Geometry check sheet. Reference: the model listing, model coordinates, mm. A direction names the side the tool comes from. Coordinates: 2 decimals unless noted, no trailing zeros.
from build123d import *

# Parameters (mm, degrees)
ESQUISSE1_W                  = 20
ESQUISSE1_H                  = 18
BOSS_EXTRU_1_DEPTH           = 20
ENL_V_MAT_EXTRU_1_DEPTH      = 34.526109228
ENL_V_MAT_EXTRU_1_DEPTH_BACK = 34.526109228
ESQUISSE4_W                  = 23.372047651
ESQUISSE4_H                  = 17.8
ENL_V_MAT_EXTRU_3_DEPTH      = 1
CONG_2_R                     = 40
ESQUISSE5_R                  = 2.15
ENL_V_MAT_EXTRU_4_DEPTH      = 31.724582991
CONG_3_R                     = 9
CHANFREIN1_SIZE              = 20.578216064
CHANFREIN1_SIZE_2            = 4
CONG_4_R                     = 4
ESQUISSE6_R                  = 1.1
ENL_V_MAT_EXTRU_5_DEPTH      = 253.375332695
ESQUISSE10_R                 = 1.9
ENL_V_MAT_EXTRU_6_DEPTH      = 7.5


# Some blends are built 0.0001 mm under size
with BuildPart() as part:
    # Esquisse1 → Boss.-Extru.1 (new body)
    with BuildSketch(Plane.XY):
        with Locations((10, 3)):
            Rectangle(ESQUISSE1_W, ESQUISSE1_H)
    extrude(amount=BOSS_EXTRU_1_DEPTH)

    # Esquisse2 → Enlèv. mat.-Extru.1 (cut, two sides: drawn at the far end of the back side and taken through both)
    with BuildSketch(Plane(origin=(0, 12, 0), x_dir=(1, 0, 0), z_dir=(0, 1, 0)).offset(-ENL_V_MAT_EXTRU_1_DEPTH_BACK)):
        Polygon((85.451214086, 12.384445057), (20.045630921, -0.0408989), (0, -3.849042594), (0, 0), (0, 66.575366927), (71.310016401, 179.020907021), (156.761230487, 124.829985151), align=None)
    extrude(amount=ENL_V_MAT_EXTRU_1_DEPTH + ENL_V_MAT_EXTRU_1_DEPTH_BACK, mode=Mode.SUBTRACT)

    # Esquisse4 → Enlèv. mat.-Extru.3 (cut)
    with BuildSketch(Plane(origin=(0.705746644, 0, 3.714969257), x_dir=(-0.9824291803850712, 0, 0.1866357562952965), z_dir=(-0.1866357562952965, 0, -0.9824291803850712))):
        with Locations((-7.953308699, 3)):
            Rectangle(ESQUISSE4_W, ESQUISSE4_H)
    extrude(amount=-ENL_V_MAT_EXTRU_3_DEPTH, mode=Mode.SUBTRACT)

    # Congé2
    # the kernel refuses this fillet: 40 mm, written as the material it adds along each edge
    with BuildSketch(Plane(origin=(41.830053891, 11.9, -3.079684565), x_dir=(0, -1, 0), z_dir=(-0.9824291803850712, 0, 0.1866357562952965))) as cong_2_piece_1_section:
        with BuildLine():
            CenterArc((8.888194417, -40), CONG_2_R, 90, 12.838568141)
            Line((0, -1), (0, 0))
            Line((0, 0), (8.888194417, 0))
        make_face()
    cong_2_piece_1 = extrude(amount=64.798673587, mode=Mode.PRIVATE)
    cong_2_piece_1 = split(cong_2_piece_1, bisect_by=Plane(origin=(20, 11.9, -3.079684565), z_dir=(-1, 0, 0)), keep=Keep.TOP, mode=Mode.PRIVATE)
    cong_2_piece_1 = split(cong_2_piece_1, bisect_by=Plane(origin=(0, 11.9, -3.079684565), z_dir=(1, 0, 0)), keep=Keep.TOP, mode=Mode.PRIVATE)
    add(cong_2_piece_1)
    with BuildSketch(Plane(origin=(-21.830053891, -5.9, 9.014064887), x_dir=(-0.18663575629529652, 1.7763568394002434e-15, -0.9824291803850713), z_dir=(0.9824291803850712, 0, -0.1866357562952965))) as cong_2_piece_2_section:
        with BuildLine():
            CenterArc((40, 8.888194417), CONG_2_R, 180, 12.838568141)
            Line((0, 8.888194417), (0, 0))
            Line((0, 0), (1, 0))
        make_face()
    cong_2_piece_2 = extrude(amount=64.798673587, mode=Mode.PRIVATE)
    cong_2_piece_2 = split(cong_2_piece_2, bisect_by=Plane(origin=(20, -5.9, 9.014064887), z_dir=(-1, 0, 0)), keep=Keep.TOP, mode=Mode.PRIVATE)
    cong_2_piece_2 = split(cong_2_piece_2, bisect_by=Plane(origin=(0, -5.9, 9.014064887), z_dir=(1, 0, 0)), keep=Keep.TOP, mode=Mode.PRIVATE)
    add(cong_2_piece_2)

    # Esquisse5 → Enlèv. mat.-Extru.4 (cut, through all)
    with BuildSketch(Plane.ZY):
        with Locations((13.5, 3)):
            Circle(ESQUISSE5_R)
    extrude(amount=-ENL_V_MAT_EXTRU_4_DEPTH, mode=Mode.SUBTRACT)

    # Congé3
    cong_3_edges = [part.edges().sort_by_distance(p)[0] for p in [
        (10, 12, 20),
        (10, -6, 20),
    ]]
    fillet(cong_3_edges, radius=CONG_3_R - 0.0001)  # a hair under: the kernel refuses the full size

    # Chanfrein1
    # the kernel refuses this chamfer: 20.578216064, 4 mm, written as the material it takes off along each edge
    with BuildSketch(Plane(origin=(20, -6, -53.417428004), x_dir=(-1, 0, 0), z_dir=(0, 0, 1))) as chanfrein1_piece_1:
        Polygon((CHANFREIN1_SIZE, 0), (0, -CHANFREIN1_SIZE_2), (0, 0), align=None)
    extrude(amount=64.417528004, mode=Mode.SUBTRACT)
    with BuildSketch(Plane(origin=(20, 2.9999, 11.0001), x_dir=(0, -1, 0), z_dir=(0, 0, -1))) as chanfrein1_piece_2:
        Polygon((8.9999, CHANFREIN1_SIZE), (8.9999 - CHANFREIN1_SIZE_2, 0), (8.9999, 0), align=None)
    revolve(axis=Axis((20, 2.9999, 11.0001), (-1, 0, 0)), revolution_arc=90, mode=Mode.SUBTRACT)
    with BuildSketch(Plane(origin=(20, 3.0001, 11.0001), x_dir=(0, 0, 1), z_dir=(0, -1, 0))) as chanfrein1_piece_3:
        Polygon((8.9999, CHANFREIN1_SIZE), (8.9999 - CHANFREIN1_SIZE_2, 0), (8.9999, 0), align=None)
    revolve(axis=Axis((20, 3.0001, 11.0001), (-1, 0, 0)), revolution_arc=90, mode=Mode.SUBTRACT)
    with BuildSketch(Plane(origin=(20, 12, -53.417428004), x_dir=(-1, 0, 0), z_dir=(0, 0, 1))) as chanfrein1_piece_4:
        Polygon((CHANFREIN1_SIZE, 0), (0, CHANFREIN1_SIZE_2), (0, 0), align=None)
    extrude(amount=64.417528004, mode=Mode.SUBTRACT)
    with BuildSketch(Plane(origin=(20, 2.9999, 20), x_dir=(-1, 0, 0), z_dir=(0, 1, 0))) as chanfrein1_piece_5:
        Polygon((CHANFREIN1_SIZE, 0), (0, -CHANFREIN1_SIZE_2), (0, 0), align=None)
    extrude(amount=0.0002, mode=Mode.SUBTRACT)

    # Congé4
    # the kernel refuses this fillet: 4 mm, written as the material it takes off along each edge
    with BuildSketch(Plane(origin=(20, -2, -7.493740481), x_dir=(-0.9816271834478703, -0.19080899537548365, 0), z_dir=(0, 0, 1))) as cong_4_piece_1:
        with BuildLine():
            CenterArc((CONG_4_R * 0.824336385818, -CONG_4_R), CONG_4_R, 90, 79)
            Line((-CONG_4_R * 0.157290797629, -CONG_4_R * 0.809191004625), (0, 0))
            Line((0, 0), (CONG_4_R * 0.824336385818, 0))
        make_face()
    extrude(amount=18.493840481, mode=Mode.SUBTRACT)
    with BuildSketch(Plane(origin=(20, 2.9999, 11.0001), x_dir=(0, -1, 0), z_dir=(0, 0, -1))) as cong_4_piece_2:
        with BuildLine():
            CenterArc((4.9999 - CONG_4_R * 0.824336385818, CONG_4_R), CONG_4_R, 270, 79)
            Line((4.9999 - CONG_4_R * 0.824336385818, 0), (4.9999, 0))
            Line((4.9999, 0), (4.9999 + CONG_4_R * 0.157290797629, CONG_4_R * 0.809191004625))
        make_face()
    revolve(axis=Axis((20, 2.9999, 11.0001), (-1, 0, 0)), revolution_arc=90, mode=Mode.SUBTRACT)
    with BuildSketch(Plane(origin=(20, 3.0001, 11.0001), x_dir=(0, 0, 1), z_dir=(0, -1, 0))) as cong_4_piece_3:
        with BuildLine():
            CenterArc((4.9999 - CONG_4_R * 0.824336385818, CONG_4_R), CONG_4_R, 270, 79)
            Line((4.9999 - CONG_4_R * 0.824336385818, 0), (4.9999, 0))
            Line((4.9999, 0), (4.9999 + CONG_4_R * 0.157290797629, CONG_4_R * 0.809191004625))
        make_face()
    revolve(axis=Axis((20, 3.0001, 11.0001), (-1, 0, 0)), revolution_arc=90, mode=Mode.SUBTRACT)
    with BuildSketch(Plane(origin=(20, 8, -7.493740481), x_dir=(-0.9816271834478704, 0.19080899537548335, 0), z_dir=(0, 0, 1))) as cong_4_piece_4:
        with BuildLine():
            CenterArc((CONG_4_R * 0.824336385818, CONG_4_R), CONG_4_R, 191, 79)
            Line((-CONG_4_R * 0.157290797629, CONG_4_R * 0.809191004625), (0, 0))
            Line((0, 0), (CONG_4_R * 0.824336385818, 0))
        make_face()
    extrude(amount=18.493840481, mode=Mode.SUBTRACT)
    with BuildSketch(Plane(origin=(20, 2.9999, 16), x_dir=(-0.9816271834478704, 0, 0.19080899537548315), z_dir=(0, 1, 0))) as cong_4_piece_5:
        with BuildLine():
            CenterArc((CONG_4_R * 0.824336385818, -CONG_4_R), CONG_4_R, 90, 79)
            Line((-CONG_4_R * 0.157290797629, -CONG_4_R * 0.809191004625), (0, 0))
            Line((0, 0), (CONG_4_R * 0.824336385818, 0))
        make_face()
    extrude(amount=0.0002, mode=Mode.SUBTRACT)

    # Esquisse6 → Enlèv. mat.-Extru.5 (cut, through all)
    with BuildSketch(Plane(origin=(248.354172881, 0, -23.381298734), x_dir=(-0.9824291803850712, 0, 0.1866357562952965), z_dir=(-0.1866357562952965, 0, -0.9824291803850712))):
        with Locations(Location((244, 7.9, 0), (0, 0, 180))):
            Circle(ESQUISSE6_R)
        with Locations(Location((244, -1.9, 0), (0, 0, 180))):
            Circle(ESQUISSE6_R)
    extrude(amount=ENL_V_MAT_EXTRU_5_DEPTH, mode=Mode.SUBTRACT)

    # Esquisse10 → Enlèv. mat.-Extru.6 (cut)
    with BuildSketch(Plane(origin=(4.363786372, 0, 22.970470151), x_dir=(-0.9824291803850712, 0, 0.1866357562952965), z_dir=(-0.1866357562952965, 0, -0.9824291803850712))):
        with Locations((-4.4, 7.9)):
            Circle(ESQUISSE10_R)
        with Locations((-4.4, -1.9)):
            Circle(ESQUISSE10_R)
    extrude(amount=ENL_V_MAT_EXTRU_6_DEPTH, mode=Mode.SUBTRACT)


solid = part.part
1) Section check A-A on z = 13.5. Count the separate pieces of the cut face and the enclosed holes in it, and give its area (3 significant figures).
Data:
separate pieces: 2
enclosed holes: 2
area: 160 mm2
2) Depth check by flat-ended pin: pin 1 (1 mm diameter, centred on x = 3, z = 13, fed in from -Y); pin 2 (1.5 mm diameter, centred on y = 5.5, z = 14.5, fed in from +X); pin 3 (8 mm diameter, centred on x = 6, z = 3.5, fed in from -Y). Enter the tip coordinate at first touch or a pass-through.
Data:
pin 1: stops at y = -5.21
pin 2: stops at x = 19.55
pin 3: stops at y = -5.5
3) Mould release check, pull along X, two halves, no side actions. Record for faces 1 (the cylindrical face through (10.1, 6.4, 2.8)), 2 (the cylindrical face through (9.86, 3.65, 15.55)), 3 (the flat face through (8.26, 10.28, 7.15)), 4 (the flat face through (8.14, -0.96, 14.62)): +X half, -X half, draft (parallel to the pull), parting line (faces both ways), or undercut.
Data:
face 1: -X half
face 2: draft
face 3: +X half
face 4: undercut
4) Material ranges on probe 1 along Y at (x, z) = (6.5, 14.5); probe 2 along Y at (x, z) = (6, 13.5); probe 3 along Z at (x, y) = (5, 1.25), recorded low to high.
Data:
probe 1: y = -3.77 to -2.77, -1.03 to 1.1, 4.9 to 7.03, 8.77 to 9.77
probe 2: y = -4.31 to -2.4, -1.4 to 0.85, 5.15 to 7.4, 8.4 to 10.31
probe 3: z = 3.88 to 12.25, 14.75 to 18.72
5) Access from +Z, -Z, +X, -X, +Y, -Y to the whole of each face (thin tool, end or side, straight path). Record for faces 5 (the cylindrical face through (19.06, -1.28, 5.93)), 6 (the flat face through (7.313, 6.616, 14.776)).
Data:
face 5: +Z, -Z, +X, -Y
face 6: none
